The model under review builds one solid part; all positions refer to its coordinate system, in mm. A direction names the side the tool comes from. Round coordinates to 2 decimals unless told otherwise and drop trailing zeros. Write each loop counter-clockwise with the first axis right and the second up, starting at its lowest first coordinate (ties: lowest second). Pieces come first, ordered by that corner, then holes. Notation, with made-up numbers: M 81.5,-27.75 L 140.5,-27.75 A27 cw 140.5,-0.75 Z; hole C 76,-12.5 d7. An arc over 180 degrees is marked long. Write item = value, one per line. Start each with the question number.
Item 1: Take a section at B-B, the plane z = 0. Give the boundary of the cut face in (x, y), plus the area to 3 significant figures.
Item 2: The part is to be moulded in two halves that separate along X. For faces 1 (the flat face through (0, 9.22, 0)), 2 (the cylindrical face through (22.77, -1.23, -5.04)), 3 (the cylindrical face through (-9.27, 10.92, 2.67)), say which applies: +X half, -X half, draft (parallel to the pull), parting line (faces both ways), or undercut.
Item 3: To check wall thickness, follow line 1 along X through (y, z) = (-6, 1.75); line 2 along Y through (x, z) = (-7, 2.5). State the ranges of each line that lie inside material, in increasing order.
Item 4: Take a section at C-C, the plane y = 7.5. Give the boundary of the cut face in (x, z), plus the area to 3 significant figures.
Item 5: Take a section at A-A, the plane x = 22. Give the boundary of the cut face in (y, z) (3 decimals), plus the area to 3 significant figures.
Item 6: Take a section at D-D, the plane x = -16.5. Give the boundary of the cut face in (y, z).
Item 7: Tool access review of faces 4 (the flat face through (-23, 1, 0.635)), 5 (the flat face through (-20.13, -16, 0)), 6 (the flat face through (-22.7, 0, -6.4)), 7 (the flat face through (22.6, 0, -5.4)): name each direction out of +Z, -Z, +X, -X, +Y, -Y from which nothing blocks a thin tool from reaching the whole face with its end or side.
Item 8: For pin 1 Ø6 at (x, z) = (24.99, 4.97) entering from +Y; pin 2 Ø2 at (x, z) = (-24, 1.5) entering from -Y; pin 3 Ø4 at (y, z) = (-19.5, 3) entering from -X; pin 4 Ø4 at (x, z) = (24.99, -4.97) entering from -Y, all flat-tipped, find the tip position at first contact; note any pin that passes through.
from build123d import *

# Parameters (mm, degrees)
SKETCH2_W               = 40.259
SKETCH2_H               = 19.9898
TOP_OF_HOUSING_DEPTH    = 9.2202
OUTER_EDGE_OF_MOTOR_W   = 53.4416
OUTER_EDGE_OF_MOTOR_H   = 19.9898
MOUNTING_FIN_DEPTH      = 2.4892
SKETCH4_R               = 2.2225
MOUNTING_HOLES_DEPTH    = 30.981848954
SKETCH5_R               = 2.799999988
C24T_SPLINE_DEPTH       = 3.4544
SKETCH2_2_W             = 40.259
SKETCH2_2_H             = 19.9898
BOTTOM_OF_HOUSING_DEPTH = 29.21
SKETCH6_W               = 6.5913
SKETCH6_H               = 1.27
NUB_DEPTH               = 1.27


with BuildPart() as part:
    # Sketch2 → Top of Housing (new body)
    with BuildSketch(Plane(origin=(0, 0, 0), x_dir=(1, 0, 0), z_dir=(0, 1, 0))):
        Rectangle(SKETCH2_W, SKETCH2_H)
    extrude(amount=TOP_OF_HOUSING_DEPTH)

    # Outer Edge of Motor → Mounting Fin (add)
    with BuildSketch(Plane(origin=(0, 0, 0), x_dir=(1, 0, 0), z_dir=(0, 1, 0))):
        Rectangle(OUTER_EDGE_OF_MOTOR_W, OUTER_EDGE_OF_MOTOR_H)
    extrude(amount=-MOUNTING_FIN_DEPTH)

    # Sketch4 → Mounting Holes (cut, through all)
    with BuildSketch(Plane(origin=(0, 0, 0), x_dir=(1, 0, 0), z_dir=(0, 1, 0))):
        with Locations((-24.992246486, 4.9657)):
            Circle(SKETCH4_R)
        with Locations((-24.992246486, -4.9657)):
            Circle(SKETCH4_R)
        with Locations((24.992246486, -4.9657)):
            Circle(SKETCH4_R)
        with Locations((24.992246486, 4.9657)):
            Circle(SKETCH4_R)
    extrude(amount=-MOUNTING_HOLES_DEPTH, mode=Mode.SUBTRACT)

    # Sketch5 → C24T Spline (add)
    with BuildSketch(Plane(origin=(0, 9.2202, 0), x_dir=(1, 0, 0), z_dir=(0, 1, 0))):
        with Locations(Location((-10.1092, 0, 0), (0, 0, 270))):
            Circle(SKETCH5_R)
    extrude(amount=C24T_SPLINE_DEPTH)

    # Sketch2_2 → Bottom of Housing (add)
    with BuildSketch(Plane(origin=(0, 0, 0), x_dir=(1, 0, 0), z_dir=(0, 1, 0))):
        Rectangle(SKETCH2_2_W, SKETCH2_2_H)
    extrude(amount=-BOTTOM_OF_HOUSING_DEPTH)

    # Sketch6 → Nub (add)
    with BuildSketch(Plane(origin=(0, 0, 0), x_dir=(1, 0, 0), z_dir=(0, 1, 0))):
        with Locations((23.42515, 0)):
            Rectangle(SKETCH6_W, SKETCH6_H)
        with Locations((-23.42515, 0)):
            Rectangle(SKETCH6_W, SKETCH6_H)
    extrude(amount=NUB_DEPTH)


solid = part.part
Response values:
q1.outline = M -26.72,-2.49 L -20.13,-2.49 L -20.13,-29.21 L 20.13,-29.21 L 20.13,-2.49 L 26.72,-2.49 L 26.72,1.27 L 20.13,1.27 L 20.13,9.22 L -7.31,9.22 L -7.31,12.67 L -12.91,12.67 L -12.91,9.22 L -20.13,9.22 L -20.13,1.27 L -26.72,1.27 Z
q1.area = 1,620 mm2
q2.face_1 = draft
q2.face_2 = undercut
q2.face_3 = parting line
q3.line_1 = -20.13 to 20.13
q3.line_2 = -29.21 to 9.22
q4.outline = M -20.13,-9.99 L 20.13,-9.99 L 20.13,9.99 L -20.13,9.99 Z
q4.area = 805 mm2
q5.outline = M -2.489,-9.995 L 0,-9.995 L 0,-0.635 L 1.27,-0.635 L 1.27,0.635 L 0,0.635 L 0,9.995 L -2.489,9.995 Z
q5.area = 51.4 mm2
q6.outline = M -29.21,-9.99 L 9.22,-9.99 L 9.22,9.99 L -29.21,9.99 Z
q7.face_4 = +Z, -X, +Y
q7.face_5 = +Z, -Z, -X, -Y
q7.face_6 = -Z, -X, +Y
q7.face_7 = -Z, +X, +Y
q8.pin_1 = 0
q8.pin_2 = -2.49
q8.pin_3 = -20.13
q8.pin_4 = through
